For this review, take the finished solid that the model builds, in its own axes (mm). A direction names the side the tool comes from. Give positions to 0.01 mm unless a question says otherwise; leave off trailing zeros. Write each loop counter-clockwise with the first axis right and the second up, starting at its lowest first coordinate (ties: lowest second). Pieces come first, ordered by that corner, then holes. Notation, with made-up numbers: M 23,20.25 L 51,20.25 A22 ccw 51,38.25 Z; hole C -18,-36 d7. An arc over 180 degrees is marked long. One line per item, written item: value. Start each with the question number.
Item 1: Mouldability with a two-part tool opening along X and no side actions: class faces 4 (the face through (0.616, 0.986, 1.088)), 5 (the face through (0.585, 1.479, 2.636)), 6 (the face through (-1.2, 3, -1.2)) as released by +X, released by -X, zero draft, split by the parting line, or undercut.
Item 2: Tool access review of faces 1 (the face through (-1.25, 1, 0)), 2 (the face through (0, 17, 0)), 3 (the face through (-1.5, 9.9, 0.07)): name each direction out of +Z, -Z, +X, -X, +Y, -Y from which nothing blocks a thin tool from reaching the whole face with its end or side.
Item 3: Consider section C-C, the plane x = -2.25. Write out the cut boundary in (y, z).
Item 4: Consider section B-B, the plane y = 12. Write out the cut boundary in (x, z).
Item 5: To check wall thickness, follow probe 1 along Y at (x, z) = (1.1, 1.45); probe 2 along Y at (x, z) = (0.75, 0.15); probe 3 along X at (y, z) = (1.5, 0.2). State the ranges of each line that lie inside material, in increasing order.
Item 6: Consider section D-D, the plane y = 2.75. Write out the cut boundary in (x, z).
Item 7: Clearance check with flat-ended pins moving along their axes: pin 1 Ø1.5 at (x, y) = (-1, 10) entering from -Z; pin 2 Ø0.8 at (x, z) = (-0.5, 0) entering from -Y. State where each tip first meets the part, or that it passes through.
Item 8: Consider section A-A, the plane z = 0. Write out the cut boundary in (x, y).
Autodesk Inventor part; units mm, degrees
ref_plane "YZ Plane" through (0, 0, 0) normal (1, 0, 0) x (0, 1, 0)
ref_plane "XZ Plane" through (0, 0, 0) normal (0, 1, 0) x (-1, 0, 0)
ref_plane "XY Plane" through (0, 0, 0) normal (0, 0, 1) x (1, 0, 0)
sketch "Sketch1" plane through (0, 0, 0) normal (0, 1, 0) x (-1, 0, 0)
  circle A0 centre (0, 0) radius 2.7
  dimension "d0" = 5.4
extrude "Extrusion1" add sketch "Sketch1" along normal blind 3
sketch "Sketch2" plane through (0, 3, 0) normal (0, 1, 0) x (1, 0, 0)
  circle A0 centre (0, 0) radius 1.5
  dimension "d3" = 3
extrude "Extrusion2" add sketch "Sketch2" along normal blind 14
sketch "Sketch3" plane through (0, 0, 0) normal (0, -1, 0) x (1, 0, 0)
  line L0 (0, -1.4434) -> (-1.25, -0.7217)
  line L1 (-1.25, -0.7217) -> (-1.25, 0.7217)
  line L2 (-1.25, 0.7217) -> (0, 1.4434)
  line L3 (0, 1.4434) -> (1.25, 0.7217)
  line L4 (1.25, 0.7217) -> (1.25, -0.7217)
  line L5 (1.25, -0.7217) -> (0, -1.4434)
  point P0 (0, 0)
  point P1 (0, 0)
  dimension "d6" = 2.5
extrude "Extrusion3" cut sketch "Sketch3" against normal blind 2
properties part number "m3_bolt_14mm" material "Stainless Steel"
Model answer:
1. face 4: undercut
1. face 5: split by the parting line
1. face 6: zero draft
2. face 1: -Y
2. face 2: +Z, -Z, +X, -X, +Y
2. face 3: +Y
3. outline: M 0,-1.49 L 3,-1.49 L 3,1.49 L 0,1.49 Z
4. outline: C 0,0 d3
5. probe 1: y = 0 to 3
5. probe 2: y = 2 to 17
5. probe 3: x = -2.69 to -1.25, 1.25 to 2.69
6. outline: C 0,0 d5.4
7. pin 1: stops at z = -1.48
7. pin 2: stops at y = 2
8. outline: M -2.7,0 L -1.25,0 L -1.25,2 L 1.25,2 L 1.25,0 L 2.7,0 L 2.7,3 L 1.5,3 L 1.5,17 L -1.5,17 L -1.5,3 L -2.7,3 Z
